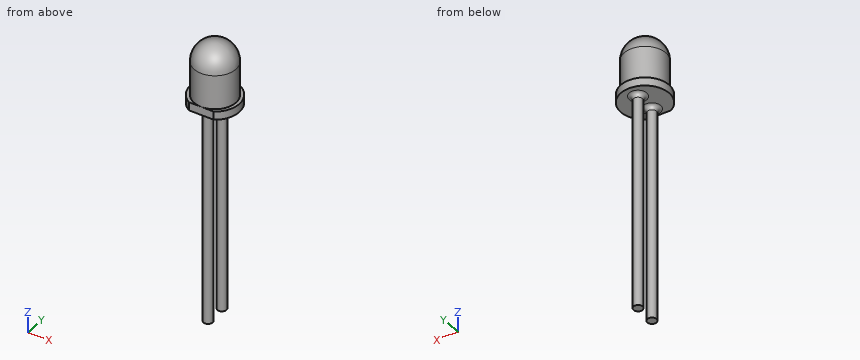
from build123d import *

# Parameters (mm, degrees)
SKETCH2_R           = 0.545
BOSS_EXTRUDE1_DEPTH = 26
SKETCH3_W           = 21.745407095
SKETCH3_H           = 16.160983483
CUT_EXTRUDE1_DEPTH  = 660
FILLET1_R           = 0.5


with BuildPart() as part:
    # Sketch1 → Revolve1 (revolve)
    with BuildSketch(Plane(origin=(0, 0, 0), x_dir=(0, 0, -1), z_dir=(1, 0, 0)), mode=Mode.PRIVATE) as revolve1_sk:
        with BuildLine():
            Line((6.6, 2.5), (2.5, 2.5))
            ThreePointArc((2.5, 2.5), (0.732233047, 1.767766953), (0, 0))
            Line((0, 0), (6.6, 0))
            Line((6.6, 0), (6.6, 2.5))
        make_face()
        Polygon((6.6, 2.9), (6.6, 2.5), (6.6, 0), (7.6, 0), (7.6, 2.780651434), (7.6, 2.9), align=None)
    revolve(revolve1_sk.sketch.rotate(Axis((0, 0, 0), (0, 0, -1)), 90), axis=Axis((0, 0, 0), (0, 0, -1)))

    # Sketch2 → Boss-Extrude1 (add)
    with BuildSketch(Plane(origin=(0, 0, -7.6), x_dir=(-1, 0, 0), z_dir=(0, 0, -1))):
        with Locations((0, 1.27)):
            Circle(SKETCH2_R)
        with Locations((0, -1.27)):
            Circle(SKETCH2_R)
    extrude(amount=BOSS_EXTRUDE1_DEPTH)

    # Sketch3 → Cut-Extrude1 (cut)
    with BuildSketch(Plane(origin=(0, -2.5, 0), x_dir=(-1, 0, 0), z_dir=(0, -1, 0))):
        with Locations((-4.780605062, 11.08865767)):
            Rectangle(SKETCH3_W, SKETCH3_H)
    extrude(amount=CUT_EXTRUDE1_DEPTH, mode=Mode.SUBTRACT)

    # Fillet1
    fillet1_edges = [part.edges().sort_by_distance(p)[0] for p in [
        (0.545, 1.27, -7.6),
        (0.545, -1.27, -7.6),
    ]]
    fillet(fillet1_edges, radius=FILLET1_R)


solid = part.part
Can you work these out from the model? Positions are in its coordinate system, mm. Round coordinates to 2 decimals unless told otherwise and drop trailing zeros. Loops run counter-clockwise (first coordinate to the right, second up) from the corner with the lowest first, then second, coordinate; pieces in that order, holes last. Notation, with made-up numbers: (56.5, -37) - (113.5, -37) arc R31 ccw to (113.5, -5) - close; hole circle Ø7 at (12, -24.5). An arc over 180 degrees is marked (long way). Answer in a Markdown table with one row per item. Add a question column.
Q1. I want a section at A-A on z = -23. List the corners of the cut face in (x, y) for me (3 decimals).
Q2. I need wall thicknesses on L1, parallel to Z at x = -1.45, y = -2.15; L2, parallel to Z at x = 2.2, y = 0.6; L3, parallel to Y at x = -0.45, z = -11.5. Which ranges of each line are inside material? Lowest first, please.
Q3. I want a section at C-C on x = -1.8. List the corners of the cut face in (y, z) for me.
Q4. I want a section at B-B on y = 1.27. List the corners of the cut face in (x, z) for me (3 decimals).
Q5. For pin 1 Ø1 at (x, y) = (-0.5, 1) entering from +Z, with a flat end and sliding along its axis, tell me the tip position at first contact or that it passes through.
A:
| question | item | result |
|---|---|---|
| 1 | outline | circle Ø1.09 at (0, -1.27); circle Ø1.09 at (0, 1.27) |
| 2 | L1 | -7.6 to -6.6 |
| 2 | L2 | -7.6 to -1.48 |
| 2 | L3 | -1.58 to -0.96, 0.96 to 1.58 |
| 3 | outline | (-2.27, -7.6) - (2.27, -7.6) - (2.27, -6.6) - (1.73, -6.6) - (1.73, -2.5) arc R1.73 ccw to (-1.73, -2.5) - (-1.73, -6.6) - (-2.27, -6.6) - close |
| 4 | outline | (-2.607, -7.6) - (-1.045, -7.6) arc R0.5 cw to (-0.545, -8.1) - (-0.545, -33.6) - (0.545, -33.6) - (0.545, -8.1) arc R0.5 cw to (1.045, -7.6) - (2.607, -7.6) - (2.607, -6.6) - (2.153, -6.6) - (2.153, -2.5) arc R2.153 ccw to (-2.153, -2.5) - (-2.153, -6.6) - (-2.607, -6.6) - close |
| 5 | pin 1 | z = -0.08 |
